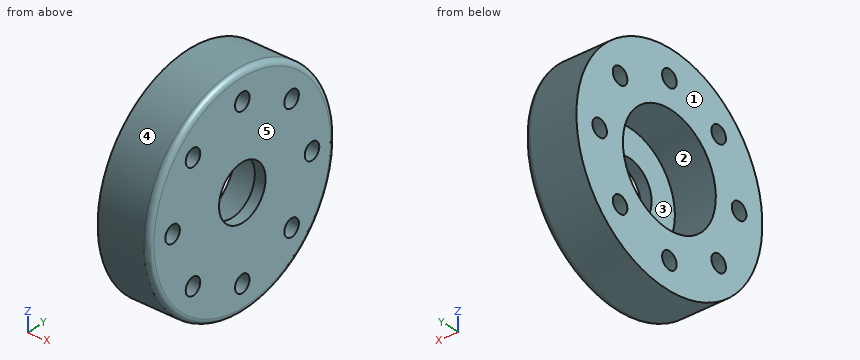
from build123d import *

# Parameters (mm, degrees)
SKETCH1_R           = 50.8
BOSS_EXTRUDE1_DEPTH = 24.511
FILLET1_R           = 2.54
SKETCH3_R           = 3.96875
CUT_EXTRUDE2_DEPTH  = 24.511
CIRPATTERN1_COUNT   = 8
SKETCH6_R           = 25.4
CUT_EXTRUDE5_DEPTH  = 19.431
SKETCH7_R           = 12.7
CUT_EXTRUDE6_DEPTH  = 5.08


with BuildPart() as part:
    # Sketch1 → Boss-Extrude1 (new body)
    with BuildSketch(Plane(origin=(0, 0, 0), x_dir=(0, 0, -1), z_dir=(1, 0, 0))):
        Circle(SKETCH1_R)
    extrude(amount=BOSS_EXTRUDE1_DEPTH)

    # Fillet1
    fillet1_edges = [part.edges().sort_by_distance(p)[0] for p in [
        (24.511, 0, 50.8),
    ]]
    fillet(fillet1_edges, radius=FILLET1_R)

    # Sketch3 → Cut-Extrude2 (cut)
    with BuildSketch(Plane(origin=(24.511, 0, 0), x_dir=(0, 0, -1), z_dir=(1, 0, 0))):
        with Locations((38.1, 0)):
            Circle(SKETCH3_R)
    cut_extrude2 = extrude(amount=-CUT_EXTRUDE2_DEPTH, mode=Mode.SUBTRACT)

    # CirPattern1: Cut-Extrude2 ×8 about axis
    cirpattern1_axis = Axis((0, 0, 0), (1, 0, 0))
    for i in range(1, CIRPATTERN1_COUNT):
        add(cut_extrude2.rotate(cirpattern1_axis, i * 360 / CIRPATTERN1_COUNT), mode=Mode.SUBTRACT)

    # Sketch6 → Cut-Extrude5 (cut)
    with BuildSketch(Plane.ZY):
        Circle(SKETCH6_R)
    extrude(amount=-CUT_EXTRUDE5_DEPTH, mode=Mode.SUBTRACT)

    # Sketch7 → Cut-Extrude6 (cut)
    with BuildSketch(Plane.ZY.offset(-19.431)):
        Circle(SKETCH7_R)
    extrude(amount=-CUT_EXTRUDE6_DEPTH, mode=Mode.SUBTRACT)


solid = part.part
Could you check a few things on this model? Use its own coordinates, in mm. Face numbers are marked on the shaded views. A direction names the side the tool comes from. Coordinates: 2 decimals unless noted, no trailing zeros. Order: outer loops, then holes, each group sorted by start corner. A loop starts at its lowest first (then second) coordinate and runs counter-clockwise, first axis right, second up.
Q1. Which directions (+Z, -Z, +X, -X, +Y, -Y) give clear straight access to the entire face, cutting with the end or side of a thin tool? Please do the marked faces 1 and 2.
Q2. Suppose I cut it at A-A on z = 0. Please give me the cut outline in (x, y), and give its area (3 significant figures).
Q3. Thinking about a two-plate mould opening in Z: for the marked faces 3, 4 and 5, which applies, released by +Z, released by -Z, zero draft, split by the parting line, or undercut?
Q4. Will these pins go through, and if not, where does the flat tip stop? pin 1 (3 mm diameter, centred on x = 22, z = -3.5, fed in from -Y); pin 2 (8 mm diameter, centred on x = 9.5, y = 26.5, fed in from +Z); pin 3 (1.5 mm diameter, centred on x = 12.5, y = -20.5, fed in from +Z).
Q5. Please list where these lines run through material, in increasing order: L1, parallel to Y at x = 8.5, z = 30; L2, parallel to Z at x = 9.5, y = 2; L3, parallel to Y at x = 20, z = -29.5.
Q6. Suppose I cut it at C-C on x = 15.5. Give the number of separate pieces and of enclosed holes in the cut face, and give its area (3 significant figures).
Answer:
1. face 1: +Z, -Z, -X, +Y, -Y
1. face 2: -X
2. outline: (0, -50.8) - (21.97, -50.8) arc R2.54 ccw to (24.51, -48.26) - (24.51, -42.07) - (0, -42.07) - close; (0, -34.13) - (24.51, -34.13) - (24.51, -12.7) - (19.43, -12.7) - (19.43, -25.4) - (0, -25.4) - close; (0, 25.4) - (19.43, 25.4) - (19.43, 12.7) - (24.51, 12.7) - (24.51, 34.13) - (0, 34.13) - close; (0, 42.07) - (24.51, 42.07) - (24.51, 48.26) arc R2.54 ccw to (21.97, 50.8) - (0, 50.8) - close
2. area: 982 mm2
3. face 3: undercut
3. face 4: split by the parting line
3. face 5: zero draft
4. pin 1: stops at y = -50.76
4. pin 2: stops at z = 45.55
4. pin 3: stops at z = 46.8
5. L1: y = -41 to -29.47, -24.41 to 24.41, 29.47 to 41
5. L2: z = -50.76 to -41.53, -34.67 to -25.32, 25.32 to 34.67, 41.53 to 50.76
5. L3: y = -41.36 to -29.97, -23.91 to 23.91, 29.97 to 41.36
6. separate pieces: 1
6. enclosed holes: 9
6. area: 5,680 mm2
